```python
from build123d import *

# Parameters (mm, degrees)
AUFSATZ_LINEAR_AUSTRAGEN1_DEPTH = 130
SKIZZE2_R                       = 3.75
SCHNITT_LINEAR_AUSTRAGEN1_DEPTH = 131.766968306


with BuildPart() as part:
    # Skizze1 → Aufsatz-Linear austragen1 (new body)
    with BuildSketch(Plane(origin=(0, 0, 0), x_dir=(1, 0, 0), z_dir=(0, 1, 0))):
        with BuildLine():
            Line((2.3, 0), (10, 0))
            Line((10, 0), (10, 3))
            ThreePointArc((10, 3), (7.071067812, 10.071067812), (0, 13))
            ThreePointArc((0, 13), (-3.16227766, 12.486832981), (-6, 11))
            Line((-6, 11), (-6, 0))
            Line((-6, 0), (-2.3, 0))
            Line((-2.3, 0), (-2.3, 3))
            Line((-2.3, 3), (-3.75, 3))
            Line((-3.75, 3), (-4, 10))
            Line((-4, 10), (4, 10))
            Line((4, 10), (3.75, 3))
            Line((3.75, 3), (2.3, 3))
            Line((2.3, 3), (2.3, 0))
        make_face()
    extrude(amount=AUFSATZ_LINEAR_AUSTRAGEN1_DEPTH)

    # Skizze2 → Schnitt-Linear austragen1 (cut, through all)
    with BuildSketch(Plane(origin=(0, 0, -3), x_dir=(-1, 0, 0), z_dir=(0, 0, -1))):
        with Locations(Location((0, 14, 0), (0, 0, 270))):
            Circle(SKIZZE2_R)
    extrude(amount=SCHNITT_LINEAR_AUSTRAGEN1_DEPTH, mode=Mode.SUBTRACT)


solid = part.part
```
Could you check a few things on this model? Use its own coordinates, in mm. A direction names the side the tool comes from. Round coordinates to 2 decimals unless told otherwise and drop trailing zeros. Loops run counter-clockwise (first coordinate to the right, second up) from the corner with the lowest first, then second, coordinate; pieces in that order, holes last. Notation, with made-up numbers: (-21.5, 1.25) -> (-4.5, 1.25) arc R25 ccw to (-4.5, 20.25) -> close; hole circle Ø9 at (85.25, -30). An arc over 180 degrees is marked (long way). One line per question, with ' | ' between items.
(1) For pin 1 Ø1 at (x, y) = (3, 22) entering from -Z; pin 2 Ø1 at (y, z) = (91, -10.5) entering from +X; pin 3 Ø0.7 at (x, y) = (-3, 40) entering from -Z, each with a flat end and sliding along its axis, tell me the tip position at first contact or that it passes through.
Model answer:
pin 1: stops at z = -12.68 | pin 2: stops at x = 7.14 | pin 3: stops at z = -12.64
(2) For faces 1 (the face through (-6, 64, -6)), 2 (the face through (-2.3, 64, -1)), which set-ups out of +Z, -Z, +X, -X, +Y, -Y let a thin tool reach every point of the face, with its end or its side?
Model answer:
face 1: +Z, -Z, -X, +Y, -Y | face 2: +Z, +Y, -Y
(3) If I drill on probe 1 along X at (y, z) = (61, -0.75); probe 2 along X at (y, z) = (88.5, -3.5); probe 3 along Y at (x, z) = (-3, -11), over which ranges is the centre line in solid material (lowest first)?
Model answer:
probe 1: x = -6 to -2.3, 2.3 to 10 | probe 2: x = -6 to -3.77, 3.77 to 9.99 | probe 3: y = 0 to 11.75, 16.25 to 130
(4) Thinking about a two-plate mould opening in X: for faces 3 (the face through (6, 64, 0)), 4 (the face through (-3.16, 11.98, -11.48)), 5 (the face through (10, 64, -1)), 6 (the face through (2.3, 64, -2)), which applies, released by +X, released by -X, zero draft, split by the parting line, or undercut?
Model answer:
face 3: zero draft | face 4: undercut | face 5: released by +X | face 6: undercut
(5) If we section it at B-B on z = -6.5: List the corners of the cut face in (x, y) for me (1 decimal), and give its area (3 significant figures).
Model answer:
outline: (-6, 0) -> (-3.9, 0) -> (-3.9, 130) -> (-6, 130) -> close; (3.9, 0) -> (9.4, 0) -> (9.4, 130) -> (3.9, 130) -> close | area: 990 mm^2
(6) If we section it at A-A on y = 92: List the corners of the cut face in (x, z) for me.
Model answer:
outline: (-6, -11) arc R10 ccw to (10, -3) -> (10, 0) -> (2.3, 0) -> (2.3, -3) -> (3.75, -3) -> (4, -10) -> (-4, -10) -> (-3.75, -3) -> (-2.3, -3) -> (-2.3, 0) -> (-6, 0) -> close
(7) If we section it at C-C on y = 14: List the corners of the cut face in (x, z) for me.
Model answer:
outline: (-6, -11) arc R10 ccw to (-3.75, -12.27) -> (-3.75, -10) -> (-4, -10) -> (-3.75, -3) -> (-2.3, -3) -> (-2.3, 0) -> (-6, 0) -> close; (2.3, -3) -> (3.75, -3) -> (4, -10) -> (3.75, -10) -> (3.75, -12.27) arc R10 ccw to (10, -3) -> (10, 0) -> (2.3, 0) -> close
